from build123d import *

# Parameters (mm, degrees)
F1_DEPTH = 25.4


with BuildPart() as f1:
    # F0 (on Front) → F1 (new body)
    with BuildSketch(Plane.XZ):
        with BuildLine():
            Line((-29.21, 0), (0, 0))
            Line((0, 0), (0, 8.128))
            Line((0, 8.128), (-6.604, 8.128))
            Line((-6.604, 8.128), (-6.604, 4.318))
            ThreePointArc((-6.604, 4.318), (-7.32242, 4.61558), (-7.62, 5.334))
            Line((-7.62, 5.334), (-7.62, 8.636))
            ThreePointArc((-7.62, 8.636), (-7.991974, 9.534026), (-8.89, 9.906))
            Line((-8.89, 9.906), (-26.67, 9.906))
            ThreePointArc((-26.67, 9.906), (-28.466051, 9.162051), (-29.21, 7.366))
            Line((-29.21, 7.366), (-29.21, 0))
        make_face()
        with BuildLine():
            Line((0, 8.128), (0, 0))
            Line((0, 0), (29.21, 0))
            Line((29.21, 0), (29.21, 7.366))
            ThreePointArc((29.21, 7.366), (28.466051, 9.162051), (26.67, 9.906))
            Line((26.67, 9.906), (8.89, 9.906))
            ThreePointArc((8.89, 9.906), (7.991974, 9.534026), (7.62, 8.636))
            Line((7.62, 8.636), (7.62, 5.334))
            ThreePointArc((7.62, 5.334), (7.32242, 4.61558), (6.604, 4.318))
            Line((6.604, 4.318), (6.604, 8.128))
            Line((6.604, 8.128), (0, 8.128))
        make_face()
        with BuildLine():
            Line((29.21, 0), (0, 0))
            Line((0, 0), (0, -8.128))
            Line((0, -8.128), (6.604, -8.128))
            Line((6.604, -8.128), (6.604, -4.318))
            ThreePointArc((6.604, -4.318), (7.32242, -4.61558), (7.62, -5.334))
            Line((7.62, -5.334), (7.62, -8.636))
            ThreePointArc((7.62, -8.636), (7.991974, -9.534026), (8.89, -9.906))
            Line((8.89, -9.906), (26.67, -9.906))
            ThreePointArc((26.67, -9.906), (28.466051, -9.162051), (29.21, -7.366))
            Line((29.21, -7.366), (29.21, 0))
        make_face()
        with BuildLine():
            Line((0, -8.128), (0, 0))
            Line((0, 0), (-29.21, 0))
            Line((-29.21, 0), (-29.21, -7.366))
            ThreePointArc((-29.21, -7.366), (-28.466051, -9.162051), (-26.67, -9.906))
            Line((-26.67, -9.906), (-8.89, -9.906))
            ThreePointArc((-8.89, -9.906), (-7.991974, -9.534026), (-7.62, -8.636))
            Line((-7.62, -8.636), (-7.62, -5.334))
            ThreePointArc((-7.62, -5.334), (-7.32242, -4.61558), (-6.604, -4.318))
            Line((-6.604, -4.318), (-6.604, -8.128))
            Line((-6.604, -8.128), (0, -8.128))
        make_face()
    extrude(amount=F1_DEPTH)


solid = f1.part
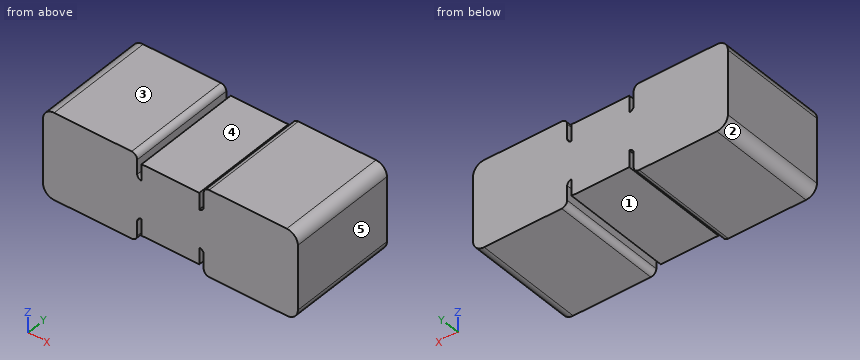
CAD build for the part. Positions are in the model's coordinates, mm. Face numbers are marked on the shaded views. A direction names the side the tool comes from. Round coordinates to 2 decimals unless told otherwise and drop trailing zeros. Write each loop counter-clockwise with the first axis right and the second up, starting at its lowest first coordinate (ties: lowest second). Pieces come first, ordered by that corner, then holes.
(1) Probe line 1 along X through (y, z) = (-10, -7.5); line 2 along X through (y, z) = (-21.75, 8); line 3 along Z through (x, y) = (-6, -22.75). List the from-to ranges inside material, lowest first.
(2) 3-axis set-ups, long thin cutter, end or side, ignore diameter. For the marked faces 1 and 2: which of +Z, -Z, +X, -X, +Y, -Y reach the whole face in a straight line?
(3) Slice it at B-B, the plane x = 5.5. Write the cut outline in (y, z).
(4) Drop flat-ended pins along their axis: P1, Ø4, axis at x = -2.5, y = -16.5, coming from the +Z side; P2, Ø4, axis at x = -2, y = -8, coming from the -Z side. Give the stop position or say it passes through.
(5) Mould opens along X. For the marked faces 3, 4 and 5 say: pulls with the +X half, pulls with the -X half, needs draft (parallel to the pull), parting line crosses it, or undercut.
(6) Slice it at A-A, the plane y = -21.5. Write the cut outline in (x, z).
From the geometry:
1. line 1: x = -29.21 to -7.62, -6.6 to 6.6, 7.62 to 29.21
1. line 2: x = -29.13 to -7.62, -6.6 to 6.6, 7.62 to 29.13
1. line 3: z = -8.13 to 8.13
2. face 1: -Z, +Y, -Y
2. face 2: -Z, -X, +Y, -Y
3. outline: (-25.4, -8.13) - (0, -8.13) - (0, 8.13) - (-25.4, 8.13) - close
4. P1: stops at z = 8.13
4. P2: stops at z = -8.13
5. face 3: needs draft
5. face 4: undercut
5. face 5: pulls with the +X half
6. outline: (-29.21, -7.37) arc R2.54 ccw to (-26.67, -9.91) - (-8.89, -9.91) arc R1.27 ccw to (-7.62, -8.64) - (-7.62, -5.33) arc R1.02 cw to (-6.6, -4.32) - (-6.6, -8.13) - (6.6, -8.13) - (6.6, -4.32) arc R1.02 cw to (7.62, -5.33) - (7.62, -8.64) arc R1.27 ccw to (8.89, -9.91) - (26.67, -9.91) arc R2.54 ccw to (29.21, -7.37) - (29.21, 7.37) arc R2.54 ccw to (26.67, 9.91) - (8.89, 9.91) arc R1.27 ccw to (7.62, 8.64) - (7.62, 5.33) arc R1.02 cw to (6.6, 4.32) - (6.6, 8.13) - (-6.6, 8.13) - (-6.6, 4.32) arc R1.02 cw to (-7.62, 5.33) - (-7.62, 8.64) arc R1.27 ccw to (-8.89, 9.91) - (-26.67, 9.91) arc R2.54 ccw to (-29.21, 7.37) - close
